Read the model definition and answer for the solid it produces. Units are mm, in the model's axes. A direction names the side the tool comes from. Give positions to 0.01 mm unless a question says otherwise; leave off trailing zeros. Write each loop counter-clockwise with the first axis right and the second up, starting at its lowest first coordinate (ties: lowest second). Pieces come first, ordered by that corner, then holes. Notation, with made-up numbers: (62, 51.5) -> (94, 51.5) arc R38 ccw to (94, 89.5) -> close; hole circle Ø11 at (14, -37.75). An arc over 180 degrees is marked (long way). Use a Markdown table: item, result.
from build123d import *

# Parameters (mm, degrees)
SKETCH_R     = 5
SKETCH_W     = 11
SKETCH_H     = 5
SKETCH_W_2   = 5
SKETCH_H_2   = 11
PAD_DEPTH    = 10
SKETCH001_R  = 11.1
POCKET_DEPTH = 8


with BuildPart() as part:
    # Sketch → Pad (new body)
    with BuildSketch(Plane.XY):
        Polygon((29.698485, 0), (0, 29.698485), (-29.698485, 0), (0, -29.698485), align=None)
        Circle(SKETCH_R, mode=Mode.SUBTRACT)
        with Locations((-18.5, 0)):
            Rectangle(SKETCH_W, SKETCH_H, mode=Mode.SUBTRACT)
        with Locations((0, 18.5)):
            Rectangle(SKETCH_W_2, SKETCH_H_2, mode=Mode.SUBTRACT)
        with Locations((0, -18.5)):
            Rectangle(SKETCH_W_2, SKETCH_H_2, mode=Mode.SUBTRACT)
        with Locations((18.5, 0)):
            Rectangle(SKETCH_W, SKETCH_H, mode=Mode.SUBTRACT)
    extrude(amount=PAD_DEPTH)

    # Sketch001 → Pocket (cut)
    with BuildSketch(Plane.XY.offset(10)):
        Circle(SKETCH001_R)
    extrude(amount=-POCKET_DEPTH, mode=Mode.SUBTRACT)


solid = part.part
Item 1: Straight lines are drawn through the part: line 1 along X through (y, z) = (-22, 4.75); line 2 along Y through (x, z) = (-2, 4); line 3 along Y through (x, z) = (-20.5, 7.5). For each, find the intervals that lie inside material, in ascending order. Write a range as [from, to].
Return value:
| item | result |
|---|---|
| line 1 | [-7.7, -2.5], [2.5, 7.7] |
| line 2 | [-27.7, -24], [-13, -10.92], [10.92, 13], [24, 27.7] |
| line 3 | [-9.2, -2.5], [2.5, 9.2] |
Item 2: A tool of negligible diameter and unlimited length cuts with its end or side. For faces 1 (the face through (5.97, 9.36, 6.06)), 2 (the face through (-19, 2.5, 5)), 3 (the face through (-7, 9, 10)), from which of +Z, -Z, +X, -X, +Y, -Y can it reach the whole face along a straight path? Write none if from no direction.
Return value:
| item | result |
|---|---|
| face 1 | +Z |
| face 2 | +Z, -Z |
| face 3 | +Z, +X, -X, +Y, -Y |
Item 3: For a pull along X with two mould halves and no side action, classify faces 4 (the face through (-15.1, -14.6, 4.9)), 5 (the face through (15.1, 14.6, 4.9)), 6 (the face through (24, 0, 5)), 7 (the face through (6, 0, 0)) as +X half, -X half, draft (parallel to the pull), parting line (faces both ways), or undercut.
Return value:
| item | result |
|---|---|
| face 4 | -X half |
| face 5 | +X half |
| face 6 | undercut |
| face 7 | draft |
Item 4: A cutting plane is placed at D-D (y = 6). Give the vertices of the cut face in (x, z).
Return value:
| item | result |
|---|---|
| outline | (-23.7, 0) -> (23.7, 0) -> (23.7, 10) -> (9.34, 10) -> (9.34, 2) -> (-9.34, 2) -> (-9.34, 10) -> (-23.7, 10) -> close |
Item 5: Each of these flat-tipped pins is pushed along its axis until it touches: P1, Ø5, axis at x = -16.5, z = 4, coming from the +Y side; P2, Ø3, axis at x = -16, z = 7, coming from the -Y side; P3, Ø2.5, axis at y = 0.5, z = 6.5, coming from the -X side. Where does it stop, or does it pass through?
Return value:
| item | result |
|---|---|
| P1 | y = 15.7 |
| P2 | y = -15.2 |
| P3 | x = -29.7 |
Item 6: A cutting plane is placed at A-A (z = 8). Give the vertices of the cut face in (x, y), then the cut area to 3 significant figures.
Return value:
| item | result |
|---|---|
| outline | (-29.7, 0) -> (0, -29.7) -> (29.7, 0) -> (0, 29.7) -> close; hole (-24, -2.5) -> (-13, -2.5) -> (-13, 2.5) -> (-24, 2.5) -> close; hole circle Ø22.2 at (0, 0); hole (-2.5, -24) -> (2.5, -24) -> (2.5, -13) -> (-2.5, -13) -> close; hole (-2.5, 13) -> (2.5, 13) -> (2.5, 24) -> (-2.5, 24) -> close; hole (13, -2.5) -> (24, -2.5) -> (24, 2.5) -> (13, 2.5) -> close |
| area | 1,160 mm^2 |
Item 7: A cutting plane is placed at B-B (x = -18.5). Give the vertices of the cut face in (y, z).
Return value:
| item | result |
|---|---|
| outline | (-11.2, 0) -> (-2.5, 0) -> (-2.5, 10) -> (-11.2, 10) -> close; (2.5, 0) -> (11.2, 0) -> (11.2, 10) -> (2.5, 10) -> close |
Item 8: A cutting plane is placed at C-C (y = -17). Give the vertices of the cut face in (x, z).
Return value:
| item | result |
|---|---|
| outline | (-12.7, 0) -> (-2.5, 0) -> (-2.5, 10) -> (-12.7, 10) -> close; (2.5, 0) -> (12.7, 0) -> (12.7, 10) -> (2.5, 10) -> close |
